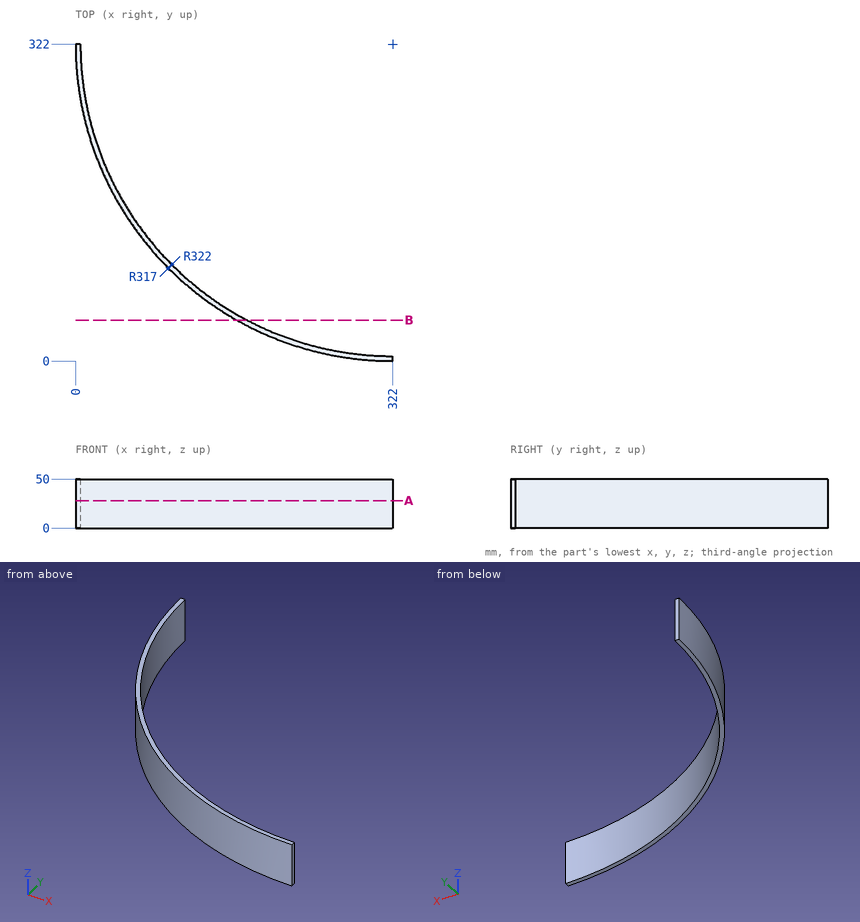
Could you check a few things on this drawing? It's one solid part, dimensions in mm from its lowest x, y, z. Give positions to 0.01 mm unless a question says otherwise; leave off trailing zeros. Order: outer loops, then holes, each group sorted by start corner. A loop starts at its lowest first (then second) coordinate and runs counter-clockwise, first axis right, second up. Notation, with made-up numbers: (29.5, 62.25) - (69.5, 62.25) arc R24 cw to (69.5, 95.25) - close; hole circle Ø8 at (12, 23.25). An arc over 180 degrees is marked (long way). One line per item, written item: value. Start each with the question number.
1. Imagine slicing it at A-A on z = 28. List the corners of the cut face in (x, y) for me, plus the area to 3 significant figures.
2. If I drill on probe 1 along Y at (x, z) = (301, 26.5); probe 2 along X at (y, z) = (227.5, 38); probe 3 along X at (y, z) = (202.5, 33.5), over which ranges is the centre line in solid material (lowest first)?
3. Imagine slicing it at B-B on y = 41.5. List the corners of the cut face in (x, z) for me, plus the area to 3 significant figures.
4. For P1, Ø10, axis at x = 120, z = 10, coming from the -Y side; P2, Ø3, axis at x = 116.5, z = 33, coming from the -Y side; P3, Ø3, axis at x = 77, z = 38, coming from the -Y side, each with a flat end and sliding along its axis, tell me the tip position at first contact or that it passes through.
Values:
1. outline: (0, 322) arc R322 ccw to (322, 0) - (322, 5) arc R317 cw to (5, 322) - close
1. area: 2,510 mm²
2. probe 1: 0.69 to 5.7
2. probe 2: 14.18 to 19.41
2. probe 3: 23 to 28.39
3. outline: (163.87, 0) - (174.32, 0) - (174.32, 50) - (163.87, 50) - close
3. area: 522 mm²
4. P1: y = 67.29
4. P2: y = 72.87
4. P3: y = 111.31
